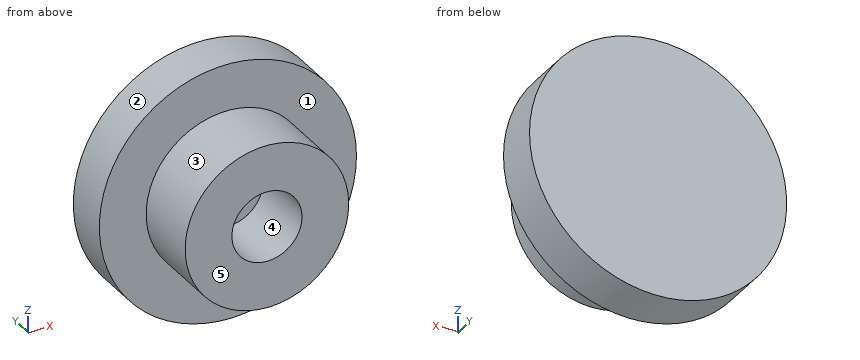
Autodesk Inventor part; units mm, degrees
ref_plane "YZ Plane" through (0, 0, 0) normal (1, 0, 0) x (0, 1, 0)
ref_plane "XZ Plane" through (0, 0, 0) normal (0, 1, 0) x (-1, 0, 0)
ref_plane "XY Plane" through (0, 0, 0) normal (0, 0, 1) x (1, 0, 0)
sketch "Sketch1" plane through (0, 0, 0) normal (0, 0, 1) x (1, 0, 0)
  line L0 (0, 0) -> (1.5, 0)
  line L1 (1.5, 0) -> (1.5, 3)
  line L2 (1.5, 3) -> (5.5, 3)
  line L3 (5.5, 3) -> (5.5, 5)
  line L4 (5.5, 5) -> (0, 5)
  line L5 (0, 5) -> (0, 3)
  line L6 (0, 3) -> (1.5, 3)
  line L7 (1.5, 0) -> (3.5, 0)
  line L8 (3.5, 0) -> (3.5, 3)
  line L9 (0, -1) -> (0, 6)
  dimension "d0" = 1.5
  dimension "d1" = 3
  dimension "d2" = 4
  dimension "d3" = 2
  dimension "d4" = 2
revolve "Revolution1" add sketch "Sketch1" angle 360 about axis through (0, -10, 0) along (0, 1, 0) contours L1 L2 L8 L7 | L5 L4 L3 L2 L6
thread "Thread1"
properties part number "FijadorParaBloqueo"
The listing builds one solid part. Answer for the finished solid, in the listing's coordinates (mm). Face numbers are marked on the shaded views. A direction names the side the tool comes from. Round coordinates to 2 decimals unless told otherwise and drop trailing zeros. Order: outer loops, then holes, each group sorted by start corner. A loop starts at its lowest first (then second) coordinate and runs counter-clockwise, first axis right, second up. Notation, with made-up numbers: (-35, 39) - (-6, 39) arc R24 ccw to (-6, 52) - close; hole circle Ø6 at (60.5, -39). An arc over 180 degrees is marked (long way). Write item = value, one per line. Start each with the question number.
1) Section A-A, the plane x = 0 is taken. Write down the section's boundary in (y, z).
2) Straight lines are drawn through the part: L1, parallel to X at y = 2.35, z = 0; L2, parallel to Y at x = 2.5, z = -3.75. For each, find the intervals that lie inside material, in ascending order.
3) For a pull along X with two mould halves and no side action, classify the marked faces 3, 4 and 5 as released by +X, released by -X, zero draft, split by the parting line, or undercut.
4) Section C-C, the plane y = 0.45 is taken. Write down the section's boundary in (x, z), plus the area to 3 significant figures.
5) Section D-D, the plane y = 3.5 is taken. Write down the section's boundary in (x, z), plus the area to 3 significant figures.
6) Section B-B, the plane z = -2.75 is taken. Write down the section's boundary in (x, y).
7) Given pin 1 (1 mm diameter, centred on y = 2, z = -2.5, fed in from +X); pin 2 (0.9 mm diameter, centred on x = -0.5, z = 0, fed in from -Y); pin 3 (2 mm diameter, centred on y = 1.5, z = -0.5, fed in from +X), each flat-ended and moving along its own axis, determine where each tip first touches the part or whether it passes through.
8) For the marked faces 1 and 2, determine the directions among +Z, -Z, +X, -X, +Y, -Y from which every point of the face is accessible in a straight line to the end or side of a thin tool.
Results list:
q1.outline = (0, -3.5) - (3, -3.5) - (3, -5.5) - (5, -5.5) - (5, 5.5) - (3, 5.5) - (3, 3.5) - (0, 3.5) - (0, 1.5) - (3, 1.5) - (3, -1.5) - (0, -1.5) - close
q2.L1 = -3.5 to -1.5, 1.5 to 3.5
q2.L2 = 3 to 5
q3.face_3 = split by the parting line
q3.face_4 = undercut
q3.face_5 = zero draft
q4.outline = circle Ø7 at (0, 0); hole circle Ø3 at (0, 0)
q4.area = 31.4 mm^2
q5.outline = circle Ø11 at (0, 0)
q5.area = 95.0 mm^2
q6.outline = (-4.76, 3) - (-2.17, 3) - (-2.17, 0) - (2.17, 0) - (2.17, 3) - (4.76, 3) - (4.76, 5) - (-4.76, 5) - close
q7.pin_1 = 2.87
q7.pin_2 = 3
q7.pin_3 = 3.5
q8.face_1 = -Y
q8.face_2 = +Y, -Y
